Autodesk Inventor part; units mm, degrees
ref_plane "YZ Plane" through (0, 0, 0) normal (1, 0, 0) x (0, 1, 0)
ref_plane "XZ Plane" through (0, 0, 0) normal (0, 1, 0) x (-1, 0, 0)
ref_plane "XY Plane" through (0, 0, 0) normal (0, 0, 1) x (1, 0, 0)
sketch "Boceto1" plane through (0, 0, 0) normal (0, 0, 1) x (1, 0, 0)
  line L0 (-275, -100) -> (275, -100)
  line L1 (275, -100) -> (275, 100)
  line L2 (275, 100) -> (-275, 100)
  line L3 (-275, 100) -> (-275, -100)
  line L4 (-275, -100) -> (275, 100) construction
  line L5 (275, -100) -> (-275, 100) construction
  point P0 (0, 0)
  dimension "ancho" = 550
  dimension "alto" = 200
extrude "Extrusión1" add sketch "Boceto1" along normal blind 18
sketch "Boceto2" plane through (0, 0, 18) normal (0, 0, 1) x (1, 0, 0)
  line L0 (247.5, -86.6667) -> (110, -86.6667)
  line L1 (110, -86.6667) -> (110, -66.6667)
  line L2 (110, -66.6667) -> (247.5, -66.6667)
  line L3 (247.5, -66.6667) -> (247.5, -86.6667)
  line L4 (275, -100) -> (275, 100)
  line L5 (-110, -86.6667) -> (-247.5, -86.6667)
  line L6 (-247.5, -86.6667) -> (-247.5, -66.6667)
  line L7 (-247.5, -66.6667) -> (-110, -66.6667)
  line L8 (-110, -66.6667) -> (-110, -86.6667)
  line L9 (-275, 100) -> (-275, -100)
  line L10 (-275, -100) -> (275, -100)
  line L11 (68.75, -86.6667) -> (-68.75, -86.6667)
  line L12 (-68.75, -86.6667) -> (-68.75, -66.6667)
  line L13 (-68.75, -66.6667) -> (68.75, -66.6667)
  line L14 (68.75, -66.6667) -> (68.75, -86.6667)
  line L15 (275, 100) -> (-275, 100)
  line L16 (247.5, 86.6667) -> (137.5, 86.6667)
  line L17 (137.5, 86.6667) -> (137.5, -46.6667)
  line L18 (137.5, -46.6667) -> (247.5, -46.6667)
  line L19 (247.5, -46.6667) -> (247.5, 86.6667)
  line L20 (-247.5, 86.6667) -> (-137.5, 86.6667)
  line L21 (-137.5, 86.6667) -> (-137.5, 31.6667)
  line L22 (-137.5, 31.6667) -> (-247.5, 31.6667)
  line L23 (-247.5, 31.6667) -> (-247.5, 86.6667)
  line L24 (-247.5, 23.8235) -> (-137.5, 23.8235)
  line L25 (-137.5, 23.8235) -> (-137.5, -31.1765)
  line L26 (-137.5, -31.1765) -> (-247.5, -31.1765)
  line L27 (-247.5, -31.1765) -> (-247.5, 23.8235)
  line L28 (-247.5, -59.0196) -> (-137.5, -59.0196)
  line L29 (-137.5, -59.0196) -> (-137.5, -39.0196)
  line L30 (-137.5, -39.0196) -> (-247.5, -39.0196)
  line L31 (-247.5, -39.0196) -> (-247.5, -59.0196)
  point P0 (0, 0)
  dimension "d4" = 137.5
  dimension "d5" = 20
  dimension "d6" = 27.5
  dimension "d7" = 137.5
  dimension "d8" = 20
  dimension "d9" = 27.5
  dimension "d10" = 13.3333
  dimension "d11" = 13.3333
  dimension "d12" = 137.5
  dimension "d13" = 41.25
  dimension "d14" = 41.25
  dimension "d15" = 20
  dimension "d17" = 110
  dimension "d18" = 133.3333
  dimension "d19" = 27.5
  dimension "d20" = 13.3333
  dimension "d21" = 110
  dimension "d22" = 55
  dimension "d23" = 27.5
  dimension "d24" = 13.3333
  dimension "d25" = 110
  dimension "d26" = 55
  dimension "d27" = 27.5
  dimension "d28" = 7.8431
  dimension "d29" = 110
  dimension "d30" = 20
  dimension "d31" = 7.8431
  dimension "d32" = 7.6471
extrude "Extrusión2" cut sketch "Boceto2" against normal blind 6 contours L0 L1 L2 L3 | L5 L6 L7 L8 | L11 L12 L13 L14 | L19 L18 L17 L16 | L20 L21 L22 L23 | L24 L25 L26 L27 | L31 L30 L29 L28
sketch "Boceto3" plane through (0, 0, 0) normal (0, 0, -1) x (-1, 0, 0)
  circle A0 centre (266, -33.3333) radius 4.5
  circle A1 centre (266, 33.3333) radius 4.5
  circle A2 centre (-266, 33.3333) radius 4.5
  circle A3 centre (-266, -33.3333) radius 4.5
  line L0 (275, 100) -> (275, -100)
  line L1 (275, -100) -> (-275, -100)
  line L2 (-275, 100) -> (275, 100)
  line L3 (-275, -100) -> (-275, 100)
  point P0 (0, 0)
  dimension "d35" = 9
  dimension "d36" = 9
  dimension "d37" = 9
  dimension "d38" = 9
  dimension "d39" = 9
  dimension "d40" = 66.6667
  dimension "d41" = 9
  dimension "d42" = 66.6667
  dimension "d43" = 9
  dimension "d44" = 66.6667
  dimension "d45" = 9
  dimension "d46" = 66.6667
extrude "Extrusión3" cut sketch "Boceto3" against normal blind 6 contours A0 | A1 | A2 | A3
sketch "Boceto4" plane through (275, -100, 0) normal (1, 0, 0) x (0, 0, -1)
  circle A0 centre (-8.4205, 125) radius 2
  circle A1 centre (-8.4205, 75) radius 2
  line L0 (0, 0) -> (-18, 0)
  point P0 (0, 100)
  point P1 (-9, 0)
  dimension "d49" = 4
  dimension "d50" = 4
  dimension "d51" = 50
  dimension "d52" = 75
extrude "Extrusión4" cut sketch "Boceto4" against normal blind 600
equation "\"d4\" = 0.25 * ancho"
equation "\"d5\" = 0.1 * alto"
equation "\"d6\" = 0.05 * ancho"
equation "\"d7\" = d4"
equation "\"d8\" = d5"
equation "\"d9\" = d6"
equation "\"d10\" = 0.0666667 * alto"
equation "\"d11\" = 0.0666667 * alto"
equation "\"d12\" = d4"
equation "\"d13\" = d14"
equation "\"d15\" = d5"
equation "\"d17\" = 0.2 * ancho"
equation "\"d18\" = 0.666667 * alto"
equation "\"d19\" = d6"
equation "\"d20\" = d10"
equation "\"d21\" = 0.2 * ancho"
equation "\"d22\" = 0.1 * ancho"
equation "\"d23\" = d9"
equation "\"d24\" = d11"
equation "\"d25\" = d21"
equation "\"d26\" = d22"
equation "\"d27\" = d23"
equation "\"d28\" = 0.0392157 * alto"
equation "\"d29\" = d21"
equation "\"d30\" = d5"
equation "\"d31\" = d28"
equation "\"d33\" = 0.333333 * grosor"
equation "\"d35\" = 0.5 * grosor"
equation "\"d36\" = d35"
equation "\"d37\" = d35"
equation "\"d38\" = d35"
equation "\"d39\" = 0.5 * grosor"
equation "\"d40\" = 0.333333 * alto"
equation "\"d41\" = d39"
equation "\"d42\" = d40"
equation "\"d43\" = d39"
equation "\"d44\" = d40"
equation "\"d45\" = d39"
equation "\"d46\" = d40"
equation "\"d47\" = 0.333333 * grosor"
properties part number "APM_003-2"
CAD build for the part. Positions are in the model's coordinates, mm. A direction names the side the tool comes from. Round coordinates to 2 decimals unless told otherwise and drop trailing zeros. Write each loop counter-clockwise with the first axis right and the second up, starting at its lowest first coordinate (ties: lowest second). Pieces come first, ordered by that corner, then holes. Notation, with made-up numbers: (29.5, 28.25) -> (63.5, 28.25) arc R28 cw to (63.5, 52.25) -> close; hole circle Ø1 at (46.5, -20.5). An arc over 180 degrees is marked (long way). Answer in a Markdown table with one row per item. Add a question column.
Item 1: Saw through at C-C, the plane x = 160. Write the cut outline in (y, z).
Item 2: Drill centre lines: line 1 (Y direction, x = 266, z = 4.1); line 2 (Y direction, x = 167.5, z = 13.5); line 3 (X direction, y = 3, z = 14.75). Where is each one in solid material? Low to high. Write a range as from..to.
Item 3: Drop flat-ended pins along their axis: pin 1 Ø5 at (x, y) = (-147, 57) entering from +Z; pin 2 Ø2.5 at (x, y) = (264, -34.5) entering from -Z. Give the stop position or say it passes through.
Item 4: Which spindle directions (+Z, -Z, +X, -X, +Y, -Y) get a long thin tool onto all of the face, cutting with end or side? Do faces 1 (the face through (261.708, 34.685, 2.958)), 2 (the face through (275, -1, 9)), 3 (the face through (-193, -3, 12)). Say none if no direction does.
Item 5: Mould opens along Y. For faces 4 (the face through (-4, 1, 0)), 5 (the face through (4, 100, 9)), 6 (the face through (261.7, -32, 3)) say: pulls with the +Y half, pulls with the -Y half, needs draft (parallel to the pull), parting line crosses it, or undercut.
Item 6: Saw through at A-A, the plane x = -179. Write the cut outline in (y, z).
Item 7: Saw through at B-B, the plane y = 46.5. Write the cut outline in (x, z), then the cut area to 3 significant figures.
Findings below:
| question | item | result |
|---|---|---|
| 1 | outline | (-100, 0) -> (100, 0) -> (100, 18) -> (86.67, 18) -> (86.67, 12) -> (-46.67, 12) -> (-46.67, 18) -> (-66.67, 18) -> (-66.67, 12) -> (-86.67, 12) -> (-86.67, 18) -> (-100, 18) -> close; hole circle Ø4 at (-25, 8.42); hole circle Ø4 at (25, 8.42) |
| 2 | line 1 | y = -100..-37.83, -28.83..28.83, 37.83..100 |
| 2 | line 2 | y = -100..-86.67, -66.67..-46.67, 86.67..100 |
| 2 | line 3 | x = -275..-247.5, -137.5..137.5, 247.5..275 |
| 3 | pin 1 | stops at z = 12 |
| 3 | pin 2 | stops at z = 6 |
| 4 | face 1 | -Z |
| 4 | face 2 | +Z, -Z, +X, +Y, -Y |
| 4 | face 3 | +Z |
| 5 | face 4 | needs draft |
| 5 | face 5 | pulls with the +Y half |
| 5 | face 6 | undercut |
| 6 | outline | (-100, 0) -> (100, 0) -> (100, 18) -> (86.67, 18) -> (86.67, 12) -> (31.67, 12) -> (31.67, 18) -> (23.82, 18) -> (23.82, 12) -> (-31.18, 12) -> (-31.18, 18) -> (-39.02, 18) -> (-39.02, 12) -> (-59.02, 12) -> (-59.02, 18) -> (-66.67, 18) -> (-66.67, 12) -> (-86.67, 12) -> (-86.67, 18) -> (-100, 18) -> close; hole circle Ø4 at (-25, 8.42); hole circle Ø4 at (25, 8.42) |
| 7 | outline | (-275, 0) -> (275, 0) -> (275, 18) -> (247.5, 18) -> (247.5, 12) -> (137.5, 12) -> (137.5, 18) -> (-137.5, 18) -> (-137.5, 12) -> (-247.5, 12) -> (-247.5, 18) -> (-275, 18) -> close |
| 7 | area | 8,580 mm^2 |
